Can you work these out from the model? Positions are in its coordinate system, mm. A direction names the side the tool comes from. Give positions to 0.01 mm unless a question says otherwise; leave off trailing zeros. Order: outer loops, then holes, each group sorted by start corner. A loop starts at its lowest first (then second) coordinate and runs counter-clockwise, first axis right, second up. Notation, with made-up numbers: (69.25, 52) - (100.25, 52) arc R13 ccw to (100.25, 74) - close; hole circle Ø5 at (-21.5, 89). An arc over 180 degrees is marked (long way). One line per question, with ' | ' between items.
```python
from build123d import *

# Parameters (mm, degrees)
SKETCH1_W                      = 84.401025
SKETCH1_H                      = 208.28
BOSS_EXTRUDE1_DEPTH            = 1.905
F_6_CLEARANCE_HOLE1_AT_2_COUNT = 2
F_6_CLEARANCE_HOLE1_AT_2_PITCH = 189.23
F_6_CLEARANCE_HOLE1_AT_3_COUNT = 2
F_6_CLEARANCE_HOLE1_AT_3_PITCH = 201.912164523
F_6_CLEARANCE_HOLE1_AT_4_COUNT = 2
F_6_CLEARANCE_HOLE1_AT_4_PITCH = 70.431025
SKETCH4_W                      = 8.466667
SKETCH4_H                      = 8.466667
BOSS_EXTRUDE2_DEPTH            = 9.525
CUT_EXTRUDE3_DEPTH             = 6.35
CHAMFER1_SIZE                  = 0.635


with BuildPart() as part:
    # Sketch1 → Boss-Extrude1 (new body)
    with BuildSketch(Plane.XY):
        Rectangle(SKETCH1_W, SKETCH1_H)
    extrude(amount=BOSS_EXTRUDE1_DEPTH)

    # Sketch3 → #6 Clearance Hole1 (revolve, cut)
    with BuildSketch(Plane(origin=(-32.6755125, 94.615, 1.905), x_dir=(0, -1, 0), z_dir=(1, 0, 0))):
        Polygon((0, 0), (0, 1.905), (2.15265, 1.905), (2.15265, 1.17475), (3.3274, 0), align=None)
    f_6_clearance_hole1 = revolve(axis=Axis((-32.6755125, 94.615, 8.255), (0, 0, -1)), mode=Mode.SUBTRACT)

    # #6 Clearance Hole1 at 2: #6 Clearance Hole1 ×2
    with Locations(*[(0, -i * F_6_CLEARANCE_HOLE1_AT_2_PITCH, 0) for i in range(1, F_6_CLEARANCE_HOLE1_AT_2_COUNT)]):
        add(f_6_clearance_hole1, mode=Mode.SUBTRACT)

    # #6 Clearance Hole1 at 3: #6 Clearance Hole1 ×2
    with Locations(*[Vector(0.34882011772903904, -0.9371896955619494, 0) * (i * F_6_CLEARANCE_HOLE1_AT_3_PITCH) for i in range(1, F_6_CLEARANCE_HOLE1_AT_3_COUNT)]):
        add(f_6_clearance_hole1, mode=Mode.SUBTRACT)

    # #6 Clearance Hole1 at 4: #6 Clearance Hole1 ×2
    with Locations(*[(i * F_6_CLEARANCE_HOLE1_AT_4_PITCH, 0, 0) for i in range(1, F_6_CLEARANCE_HOLE1_AT_4_COUNT)]):
        add(f_6_clearance_hole1, mode=Mode.SUBTRACT)

    # Sketch4 → Boss-Extrude2 (add)
    with BuildSketch(Plane(origin=(0, 0, 0), x_dir=(-1, 0, 0), z_dir=(0, 0, -1))):
        with Locations((-37.967179, 82.973333082)):
            Rectangle(SKETCH4_W, SKETCH4_H)
        with Locations((-37.967179, -8.0433335)):
            Rectangle(SKETCH4_W, SKETCH4_H)
        with Locations((-37.967179, -82.973333082)):
            Rectangle(SKETCH4_W, SKETCH4_H)
    extrude(amount=BOSS_EXTRUDE2_DEPTH)

    # Sketch5 → Cut-Extrude3 (cut)
    with BuildSketch(Plane(origin=(42.2005125, 0, 0), x_dir=(0, 0, -1), z_dir=(1, 0, 0))):
        Polygon((2.116666667, -82.973333082), (5.291666667, -79.798333082), (8.466666667, -82.973333082), (5.291666667, -86.148333082), align=None)
        Polygon((2.116666667, -8.0433335), (5.291666667, -4.8683335), (8.466666667, -8.0433335), (5.291666667, -11.2183335), align=None)
        Polygon((2.116666667, 82.973333082), (5.291666667, 86.148333082), (8.466666667, 82.973333082), (5.291666667, 79.798333082), align=None)
    extrude(amount=-CUT_EXTRUDE3_DEPTH, mode=Mode.SUBTRACT)

    # Chamfer1
    chamfer1_edges = [part.edges().sort_by_distance(p)[0] for p in [
        (35.8505125, 81.385833082, -3.704166667),
        (35.8505125, 84.560833082, -3.704166667),
        (35.8505125, 84.560833082, -6.879166667),
        (35.8505125, 81.385833082, -6.879166667),
        (42.2005125, 81.385833082, -3.704166667),
        (42.2005125, 81.385833082, -6.879166667),
        (42.2005125, 84.560833082, -6.879166667),
        (42.2005125, 84.560833082, -3.704166667),
        (35.8505125, -84.560833082, -3.704166667),
        (35.8505125, -81.385833082, -3.704166667),
        (35.8505125, -81.385833082, -6.879166667),
        (35.8505125, -84.560833082, -6.879166667),
        (42.2005125, -84.560833082, -3.704166667),
        (42.2005125, -84.560833082, -6.879166667),
        (42.2005125, -81.385833082, -6.879166667),
        (42.2005125, -81.385833082, -3.704166667),
        (42.2005125, -9.6308335, -3.704166667),
        (42.2005125, -9.6308335, -6.879166667),
        (42.2005125, -6.4558335, -6.879166667),
        (42.2005125, -6.4558335, -3.704166667),
    ]]
    chamfer(chamfer1_edges, length=CHAMFER1_SIZE)


solid = part.part
```
(1) On a 3-axis mill with a long thin cutter (end or side, diameter ignored), from which of +Z, -Z, +X, -X, +Y, -Y can I reach the whole of each face in a straight line? I mean faces 1 (the face through (38, -87.207, -5)), 2 (the face through (38, -3.81, -5)), 3 (the face through (41.879, 84.811, -7.072)). Say none if no direction works.
Answer below:
face 1: -Z, +X, -X, -Y | face 2: -Z, +X, -X | face 3: +X
(2) If I drill on line 1 (Z direction, x = 5, y = 62.5) (3 decimals), over which ranges is the centre line in solid material (lowest first)?
Answer below:
line 1: 0 to 1.905
(3) Will these pins go through, and if not, where does the flat tip stop? pin 1 (2 mm diameter, centred on y = -4, z = -7, fed in from -X); pin 2 (10 mm diameter, centred on x = -17.5, y = -79, fed in from -Z); pin 3 (3 mm diameter, centred on y = -78.5, z = -1, fed in from -X); pin 4 (1.4 mm diameter, centred on y = -82.5, z = -6, fed in from +X).
Answer below:
pin 1: x = 33.73 | pin 2: z = 0 | pin 3: x = -42.2 | pin 4: x = 35.85
(4) Imagine slicing it at B-B (y = -20.5). List the corners of the cut face in (x, z) for me (3 decimals), and give its area (3 significant figures).
Answer below:
outline: (-42.201, 0) - (42.201, 0) - (42.201, 1.905) - (-42.201, 1.905) - close | area: 161 mm^2
(5) If we mould it in two halves opening along Y, with no side actions, what happens to faces 4 (the face through (33.734, -83, -5)), 5 (the face through (38, 87.207, -5)), 6 (the face through (-34.13, 96.2, 0.37))? For each: released by +Y, released by -Y, zero draft, split by the parting line, or undercut.
Answer below:
face 4: zero draft | face 5: released by +Y | face 6: undercut
(6) Imagine slicing it at A-A (x = -1). List the corners of the cut face in (y, z) for me (3 decimals).
Answer below:
outline: (-104.14, 0) - (104.14, 0) - (104.14, 1.905) - (-104.14, 1.905) - close
